from build123d import *

# Parameters (mm, degrees)
SKETCH1_R           = 5.75
BOSS_EXTRUDE1_DEPTH = 4


with BuildPart() as part:
    # Sketch1 → Boss-Extrude1 (new body)
    with BuildSketch(Plane(origin=(0, 0, 0), x_dir=(1, 0, 0), z_dir=(0, 1, 0))):
        with BuildLine():
            Line((14.722227154, 13.97), (29.21, 13.97))
            ThreePointArc((29.21, 13.97), (33.700128061, 12.110128061), (35.56, 7.62))
            Line((35.56, 7.62), (35.56, -7.62))
            ThreePointArc((35.56, -7.62), (33.700128061, -12.110128061), (29.21, -13.97))
            Line((29.21, -13.97), (19.176579466, -13.97))
            ThreePointArc((19.176579466, -13.97), (16.831686562, -14.418815604), (14.818265951, -15.701818182))
            ThreePointArc((14.818265951, -15.701818182), (0, -21.59), (-14.818265951, -15.701818182))
            ThreePointArc((-14.818265951, -15.701818182), (-16.831686562, -14.418815604), (-19.176579466, -13.97))
            Line((-19.176579466, -13.97), (-29.21, -13.97))
            ThreePointArc((-29.21, -13.97), (-33.700128061, -12.110128061), (-35.56, -7.62))
            Line((-35.56, -7.62), (-35.56, 7.62))
            ThreePointArc((-35.56, 7.62), (-33.700128061, 12.110128061), (-29.21, 13.97))
            Line((-29.21, 13.97), (-14.722227154, 13.97))
            ThreePointArc((-14.722227154, 13.97), (-13.078726217, 13.753628997), (-11.547227154, 13.119261314))
            Line((-11.547227154, 13.119261314), (-8.995011096, 11.645738686))
            ThreePointArc((-8.995011096, 11.645738686), (-7.463512032, 11.011371003), (-5.820011096, 10.795))
            Line((-5.820011096, 10.795), (5.820011096, 10.795))
            ThreePointArc((5.820011096, 10.795), (7.463512032, 11.011371003), (8.995011096, 11.645738686))
            Line((8.995011096, 11.645738686), (11.547227154, 13.119261314))
            ThreePointArc((11.547227154, 13.119261314), (13.078726217, 13.753628997), (14.722227154, 13.97))
        make_face()
        Circle(SKETCH1_R, mode=Mode.SUBTRACT)
        with BuildLine():
            Line((-23.495, -2.667), (-29.21, -2.667))
            ThreePointArc((-29.21, -2.667), (-31.877, 0), (-29.21, 2.667))
            Line((-29.21, 2.667), (-23.495, 2.667))
            ThreePointArc((-23.495, 2.667), (-20.828, 0), (-23.495, -2.667))
        make_face(mode=Mode.SUBTRACT)
        with BuildLine():
            Line((23.495, 2.667), (29.21, 2.667))
            ThreePointArc((29.21, 2.667), (31.877, 0), (29.21, -2.667))
            Line((29.21, -2.667), (23.495, -2.667))
            ThreePointArc((23.495, -2.667), (20.828, 0), (23.495, 2.667))
        make_face(mode=Mode.SUBTRACT)
        with BuildLine():
            Line((-15.289419162, 6.517949192), (-13.089714637, 5.247949192))
            ThreePointArc((-13.089714637, 5.247949192), (-10.357663829, 5.98), (-11.089714637, 8.712050808))
            Line((-11.089714637, 8.712050808), (-13.289419162, 9.982050808))
            ThreePointArc((-13.289419162, 9.982050808), (-16.02146997, 9.25), (-15.289419162, 6.517949192))
        make_face(mode=Mode.SUBTRACT)
        with BuildLine():
            Line((13.289419162, 9.982050808), (11.089714637, 8.712050808))
            ThreePointArc((11.089714637, 8.712050808), (10.357663829, 5.98), (13.089714637, 5.247949192))
            Line((13.089714637, 5.247949192), (15.289419162, 6.517949192))
            ThreePointArc((15.289419162, 6.517949192), (16.02146997, 9.25), (13.289419162, 9.982050808))
        make_face(mode=Mode.SUBTRACT)
        with BuildLine():
            Line((2, -16.5), (2, -13.96))
            ThreePointArc((2, -13.96), (0, -11.96), (-2, -13.96))
            Line((-2, -13.96), (-2, -16.5))
            ThreePointArc((-2, -16.5), (0, -18.5), (2, -16.5))
        make_face(mode=Mode.SUBTRACT)
    extrude(amount=BOSS_EXTRUDE1_DEPTH)


solid = part.part
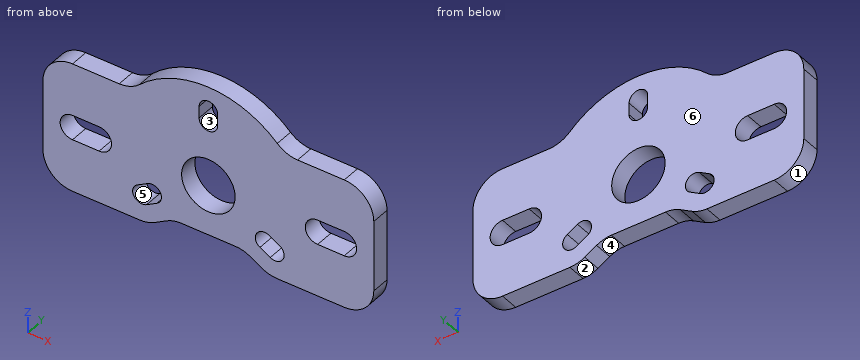
Could you check a few things on this model? Use its own coordinates, in mm. Face numbers are marked on the shaded views. A direction names the side the tool comes from. Round coordinates to 2 decimals unless told otherwise and drop trailing zeros. Order: outer loops, then holes, each group sorted by start corner. A loop starts at its lowest first (then second) coordinate and runs counter-clockwise, first axis right, second up.
Q1. Please list where these lines run through material, in increasing order: probe 1 along X at (y, z) = (2.85, 0); probe 2 along Z at (x, y) = (0, 2.2) (3 decimals); probe 3 along Z at (x, y) = (-29.5, 1.1).
Geometry says:
probe 1: x = -35.56 to -31.88, -20.83 to -5.75, 5.75 to 20.83, 31.88 to 35.56
probe 2: z = -10.795 to -5.75, 5.75 to 11.96, 18.5 to 21.59
probe 3: z = -13.96 to -2.65, 2.65 to 13.96
Q2. Thinking about a two-plate mould opening in Z: for the marked faces 4, 5 and 6, which applies, released by +Z, released by -Z, zero draft, split by the parting line, or undercut?
Geometry says:
face 4: released by -Z
face 5: undercut
face 6: zero draft
Q3. Imagine slicing it at A-A, the plane z = 0. List the corners of the cut face in (x, y) for me, then the cut area to 3 significant figures.
Geometry says:
outline: (-35.56, 0) - (-31.88, 0) - (-31.88, 4) - (-35.56, 4) - close; (-20.83, 0) - (-5.75, 0) - (-5.75, 4) - (-20.83, 4) - close; (5.75, 0) - (20.83, 0) - (20.83, 4) - (5.75, 4) - close; (31.88, 0) - (35.56, 0) - (35.56, 4) - (31.88, 4) - close
area: 150 mm2
Q4. Which directions (+Z, -Z, +X, -X, +Y, -Y) give clear straight access to the entire face, cutting with the end or side of a thin tool? Please do the marked faces 1, 2 and 3.
Geometry says:
face 1: -Z, -X, +Y, -Y
face 2: -Z, +Y, -Y
face 3: +Y, -Y
Q5. I'm going to push flat-ended pins straight in: P1, Ø10.5, axis at x = 0, z = 0, coming from the -Y side; P2, Ø6, axis at x = 27.5, z = 6.5, coming from the -Y side; P3, Ø1.2, axis at x = -26, y = 2.5, coming from the +Z side; P4, Ø0.8, axis at y = 1.5, z = 15.5, coming from the +X side. Where does each tip first touch, or does it pass through?
Geometry says:
P1: passes through
P2: stops at y = 0
P3: stops at z = 13.97
P4: stops at x = 15.56
Q6. Imagine slicing it at D-D, the plane z = 19.5. List the corners of the cut face in (x, y) for me.
Geometry says:
outline: (-9.27, 0) - (9.27, 0) - (9.27, 4) - (-9.27, 4) - close
Q7. Imagine slicing it at B-B, the plane x = 0. List the corners of the cut face in (y, z) for me (3 decimals).
Geometry says:
outline: (0, -10.795) - (4, -10.795) - (4, -5.75) - (0, -5.75) - close; (0, 5.75) - (4, 5.75) - (4, 11.96) - (0, 11.96) - close; (0, 18.5) - (4, 18.5) - (4, 21.59) - (0, 21.59) - close
Q8. Imagine slicing it at C-C, the plane y = 2.9. State how many separate pieces and enclosed holes the cut face has, then the cut area to 3 significant figures.
Geometry says:
separate pieces: 1
enclosed holes: 6
area: 1,790 mm2
